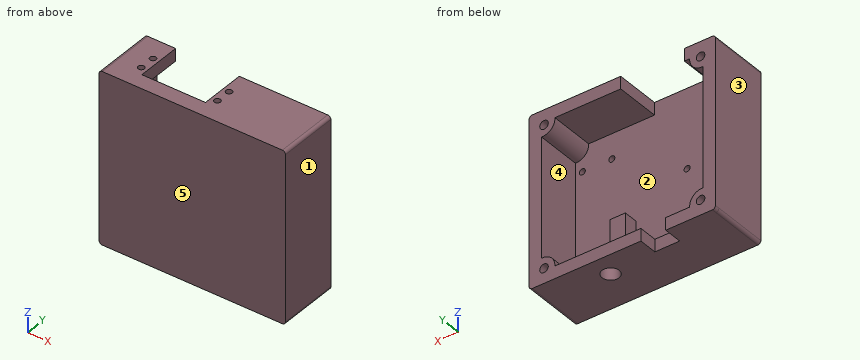
from build123d import *

# Parameters (mm, degrees)
SKETCH1_W           = 120
SKETCH1_H           = 110
BOSS_EXTRUDE1_DEPTH = 30
SKETCH2_W           = 104
SKETCH2_H           = 94
CUT_EXTRUDE1_DEPTH  = 26
FILLET1_R           = 2
CUT_EXTRUDE2_REACH  = 167.529
SKETCH3_W           = 41
SKETCH3_H           = 21
SKETCH5_R           = 2
CUT_EXTRUDE3_DEPTH  = 5
CUT_EXTRUDE4_REACH  = 167.529
SKETCH7_R           = 5.5
CUT_EXTRUDE5_REACH  = 167.529
SKETCH8_W           = 16
SKETCH8_H           = 9
SKETCH9_W           = 10
SKETCH9_H           = 32
BOSS_EXTRUDE2_DEPTH = 9
BOSS_EXTRUDE3_DEPTH = 26
BOSS_EXTRUDE4_DEPTH = 6
SKETCH11_R          = 1.95
CUT_EXTRUDE6_DEPTH  = 6
SKETCH13_R          = 2.75
CUT_EXTRUDE7_DEPTH  = 10
CUT_EXTRUDE8_REACH  = 167.529
SKETCH16_W          = 41
SKETCH16_H          = 5
BOSS_EXTRUDE5_START = 3
SKETCH21_R          = 2.75
BOSS_EXTRUDE5_DEPTH = 3


with BuildPart() as part:
    # Sketch1 → Boss-Extrude1 (new body)
    with BuildSketch(Plane(origin=(0, 0, 0), x_dir=(1, 0, 0), z_dir=(0, 1, 0))):
        with Locations((60, 55)):
            Rectangle(SKETCH1_W, SKETCH1_H)
    extrude(amount=BOSS_EXTRUDE1_DEPTH)

    # Sketch2 → Cut-Extrude1 (cut)
    with BuildSketch(Plane(origin=(0, 30, 0), x_dir=(1, 0, 0), z_dir=(0, 1, 0))):
        with Locations((60, 55)):
            Rectangle(SKETCH2_W, SKETCH2_H)
    extrude(amount=-CUT_EXTRUDE1_DEPTH, mode=Mode.SUBTRACT)

    # Fillet1
    fillet1_edges = [part.edges().sort_by_distance(p)[0] for p in [
        (112, 17, -8),
        (8, 17, -8),
        (8, 17, -102),
        (112, 17, -102),
        (0, 15, -110),
        (120, 15, -110),
        (120, 15, 0),
        (0, 15, 0),
    ]]
    fillet(fillet1_edges, radius=FILLET1_R)

    # Sketch3 → Cut-Extrude2 (cut, up to next)
    with BuildSketch(Plane.XY, mode=Mode.PRIVATE) as cut_extrude2_sk1:
        with Locations((40.5, 14.5)):
            Rectangle(SKETCH3_W, SKETCH3_H)
    cut_extrude2_tool1 = extrude(cut_extrude2_sk1.sketch, amount=-CUT_EXTRUDE2_REACH, mode=Mode.PRIVATE) & part.part
    add(cut_extrude2_tool1.solids().sort_by_distance((40.5, 14.5, 0))[0], mode=Mode.SUBTRACT)

    # Sketch5 → Cut-Extrude3 (cut)
    with BuildSketch(Plane.XY):
        with Locations((65, 8.9)):
            Circle(SKETCH5_R)
        with Locations((16, 18.9)):
            Circle(SKETCH5_R)
        with Locations((16, 8.9)):
            Circle(SKETCH5_R)
        with Locations((65, 18.9)):
            Circle(SKETCH5_R)
    extrude(amount=-CUT_EXTRUDE3_DEPTH, mode=Mode.SUBTRACT)

    # Sketch7 → Cut-Extrude4 (cut, up to next)
    with BuildSketch(Plane(origin=(0, 0, -110), x_dir=(-1, 0, 0), z_dir=(0, 0, -1)), mode=Mode.PRIVATE) as cut_extrude4_sk1:
        with Locations((-78, 19)):
            Circle(SKETCH7_R)
    cut_extrude4_tool1 = extrude(cut_extrude4_sk1.sketch, amount=-CUT_EXTRUDE4_REACH, mode=Mode.PRIVATE) & part.part
    add(cut_extrude4_tool1.solids().sort_by_distance((78, 19, -110))[0], mode=Mode.SUBTRACT)

    # Sketch8 → Cut-Extrude5 (cut, up to next)
    with BuildSketch(Plane(origin=(0, 0, -110), x_dir=(-1, 0, 0), z_dir=(0, 0, -1)), mode=Mode.PRIVATE) as cut_extrude5_sk1:
        with Locations((-40, 25.5)):
            Rectangle(SKETCH8_W, SKETCH8_H)
    cut_extrude5_tool1 = extrude(cut_extrude5_sk1.sketch, amount=-CUT_EXTRUDE5_REACH, mode=Mode.PRIVATE) & part.part
    add(cut_extrude5_tool1.solids().sort_by_distance((40, 25.5, -110))[0], mode=Mode.SUBTRACT)

    # Sketch9 → Boss-Extrude2 (add)
    with BuildSketch(Plane(origin=(0, 4, 0), x_dir=(1, 0, 0), z_dir=(0, 1, 0))):
        with Locations((78, 86)):
            Rectangle(SKETCH9_W, SKETCH9_H)
    extrude(amount=BOSS_EXTRUDE2_DEPTH)

    # Sketch10 → Boss-Extrude3 (add)
    with BuildSketch(Plane(origin=(0, 4, 0), x_dir=(1, 0, 0), z_dir=(0, 1, 0))):
        with BuildLine():
            ThreePointArc((10, 102), (8.585786438, 101.414213562), (8, 100))
            Line((8, 100), (8, 93.435688996))
            ThreePointArc((8, 93.435688996), (14.242640687, 95.757359313), (16.564311004, 102))
            Line((16.564311004, 102), (10, 102))
        make_face()
        with BuildLine():
            ThreePointArc((8, 10), (8.585786438, 8.585786438), (10, 8))
            Line((10, 8), (16.564311004, 8))
            ThreePointArc((16.564311004, 8), (14.242640687, 14.242640687), (8, 16.564311004))
            Line((8, 16.564311004), (8, 10))
        make_face()
        with BuildLine():
            ThreePointArc((110, 8), (111.414213562, 8.585786438), (112, 10))
            Line((112, 10), (112, 16.564311004))
            ThreePointArc((112, 16.564311004), (105.757359313, 14.242640687), (103.435688996, 8))
            Line((103.435688996, 8), (110, 8))
        make_face()
        with BuildLine():
            ThreePointArc((112, 100), (111.414213562, 101.414213562), (110, 102))
            Line((110, 102), (103.435688996, 102))
            ThreePointArc((103.435688996, 102), (105.757359313, 95.757359313), (112, 93.435688996))
            Line((112, 93.435688996), (112, 100))
        make_face()
    extrude(amount=BOSS_EXTRUDE3_DEPTH)

    # Sketch12 → Boss-Extrude4 (add)
    with BuildSketch(Plane.XZ):
        with BuildLine():
            Line((2, -110), (118, -110))
            ThreePointArc((118, -110), (119.414213562, -109.414213562), (120, -108))
            Line((120, -108), (120, -2))
            ThreePointArc((120, -2), (119.414213562, -0.585786438), (118, 0))
            Line((118, 0), (2, 0))
            ThreePointArc((2, 0), (0.585786438, -0.585786438), (0, -2))
            Line((0, -2), (0, -108))
            ThreePointArc((0, -108), (0.585786438, -109.414213562), (2, -110))
        make_face()
    extrude(amount=BOSS_EXTRUDE4_DEPTH)

    # Sketch11 → Cut-Extrude6 (cut)
    with BuildSketch(Plane(origin=(0, 4, 0), x_dir=(1, 0, 0), z_dir=(0, 1, 0))):
        with Locations(Location((40, 96, 0), (0, 0, 270))):
            Circle(SKETCH11_R)
        with Locations(Location((40, 51, 0), (0, 0, 270))):
            Circle(SKETCH11_R)
        with Locations(Location((88.5, 80, 0), (0, 0, 270))):
            Circle(SKETCH11_R)
        with Locations(Location((107.5, 80, 0), (0, 0, 270))):
            Circle(SKETCH11_R)
        with Locations(Location((88.5, 24, 0), (0, 0, 270))):
            Circle(SKETCH11_R)
        with Locations(Location((107.5, 24, 0), (0, 0, 270))):
            Circle(SKETCH11_R)
    extrude(amount=-CUT_EXTRUDE6_DEPTH, mode=Mode.SUBTRACT)

    # Sketch13 → Cut-Extrude7 (cut)
    with BuildSketch(Plane(origin=(0, 30, 0), x_dir=(1, 0, 0), z_dir=(0, 1, 0))):
        with Locations(Location((110.435688996, 100.435688996, 0), (0, 0, 90))):
            Circle(SKETCH13_R)
        with Locations(Location((9.564311004, 100.435688996, 0), (0, 0, 270))):
            Circle(SKETCH13_R)
        with Locations(Location((110.435688996, 9.564311004, 0), (0, 0, 270))):
            Circle(SKETCH13_R)
        with Locations(Location((9.564311004, 9.564311004, 0), (0, 0, 90))):
            Circle(SKETCH13_R)
    extrude(amount=-CUT_EXTRUDE7_DEPTH, mode=Mode.SUBTRACT)

    # Sketch16 → Cut-Extrude8 (cut, up to next)
    with BuildSketch(Plane.XY, mode=Mode.PRIVATE) as cut_extrude8_sk1:
        with Locations((40.5, 27.5)):
            Rectangle(SKETCH16_W, SKETCH16_H)
    cut_extrude8_tool1 = extrude(cut_extrude8_sk1.sketch, amount=-CUT_EXTRUDE8_REACH, mode=Mode.PRIVATE) & part.part
    add(cut_extrude8_tool1.solids().sort_by_distance((40.5, 27.5, 0))[0], mode=Mode.SUBTRACT)

    # Sketch21 → Boss-Extrude5 (add)
    # profile 1 of 2: a face of its own
    with BuildSketch(Plane(origin=(0, 30, 0), x_dir=(1, 0, 0), z_dir=(0, 1, 0)).offset(BOSS_EXTRUDE5_START)):
        with BuildLine():
            ThreePointArc((112, 16.564311004), (105.757359313, 14.242640687), (103.435688996, 8))
            Line((103.435688996, 8), (61, 8))
            Line((61, 8), (61, 0))
            Line((61, 0), (118, 0))
            ThreePointArc((118, 0), (119.414213562, 0.585786438), (120, 2))
            Line((120, 2), (120, 108))
            ThreePointArc((120, 108), (119.414213562, 109.414213562), (118, 110))
            Line((118, 110), (48, 110))
            Line((48, 110), (48, 102))
            Line((48, 102), (103.435688996, 102))
            ThreePointArc((103.435688996, 102), (105.757359313, 95.757359313), (112, 93.435688996))
            Line((112, 93.435688996), (112, 16.564311004))
        make_face()
        with Locations((110.435688996, 9.564311004)):
            Circle(SKETCH21_R, mode=Mode.SUBTRACT)
        with Locations((110.435688996, 100.435688996)):
            Circle(SKETCH21_R, mode=Mode.SUBTRACT)
    # profile 2 of 2: a face of its own
    with BuildSketch(Plane(origin=(0, 30, 0), x_dir=(1, 0, 0), z_dir=(0, 1, 0)).offset(BOSS_EXTRUDE5_START)):
        with BuildLine():
            Line((8, 16.564311004), (8, 93.435688996))
            ThreePointArc((8, 93.435688996), (14.242640687, 95.757359313), (16.564311004, 102))
            Line((16.564311004, 102), (32, 102))
            Line((32, 102), (32, 110))
            Line((32, 110), (2, 110))
            ThreePointArc((2, 110), (0.585786438, 109.414213562), (0, 108))
            Line((0, 108), (0, 2))
            ThreePointArc((0, 2), (0.585786438, 0.585786438), (2, 0))
            Line((2, 0), (20, 0))
            Line((20, 0), (20, 8))
            Line((20, 8), (16.564311004, 8))
            ThreePointArc((16.564311004, 8), (14.242640687, 14.242640687), (8, 16.564311004))
        make_face()
        with Locations((9.564311004, 9.564311004)):
            Circle(SKETCH21_R, mode=Mode.SUBTRACT)
        with Locations((9.564311004, 100.435688996)):
            Circle(SKETCH21_R, mode=Mode.SUBTRACT)
    extrude(amount=-BOSS_EXTRUDE5_DEPTH)


solid = part.part
The listing builds one solid part. Answer for the finished solid, in the listing's coordinates (mm). Face numbers are marked on the shaded views. A direction names the side the tool comes from. Give positions to 0.01 mm unless a question says otherwise; leave off trailing zeros. Write each loop counter-clockwise with the first axis right and the second up, starting at its lowest first coordinate (ties: lowest second). Pieces come first, ordered by that corner, then holes.
1) Section D-D (z = -91.5) is taken. Write down the section's boundary in (x, y).
2) Given P1, Ø6, axis at x = 40, z = -96, coming from the +Y side; P2, Ø1.5, axis at x = 25, y = 12.5, coming from the +Z side; P3, Ø2, axis at x = 65, y = 8, coming from the +Z side, each flat-ended and moving along its own axis, determine where each tip first touches the part or whether it passes through.
3) For a pull along X with two mould halves and no side action, classify the marked faces 1, 2 and 3 as pulls with the +X half, pulls with the -X half, needs draft (parallel to the pull), parting line crosses it, or undercut.
4) Section A-A (z = -24) is taken. Write down the section's boundary in (x, y).
5) Section C-C (y = 28.5) is taken. Write down the section's boundary in (x, z), and give its area (3 significant figures).
6) A tool of negligible diameter and unlimited length cuts with its end or side. For the marked faces 4 and 5, from which of +Z, -Z, +X, -X, +Y, -Y can it reach the whole face along a straight path? Write none if from no direction.
7) Find the intervals of material crossed by L1, parallel to X at y = -0.7, z = -80; L2, parallel to X at y = 0.65, z = -96; L3, parallel to Z at x = 99.5, y = 9.5, in increasing order.
8) Section B-B (x = 88.5) is taken. Write down the section's boundary in (y, z), and give its area (3 significant figures).
Response:
1. outline: (0, -6) - (120, -6) - (120, 33) - (112, 33) - (112, 4) - (83, 4) - (83, 13) - (73, 13) - (73, 4) - (8, 4) - (8, 33) - (0, 33) - close
2. P1: stops at y = 4
2. P2: stops at z = -102
2. P3: stops at z = -5
3. face 1: pulls with the +X half
3. face 2: undercut
3. face 3: pulls with the -X half
4. outline: (0, -6) - (120, -6) - (120, 33) - (112, 33) - (112, 4) - (109.45, 4) - (109.45, -2) - (105.55, -2) - (105.55, 4) - (90.45, 4) - (90.45, -2) - (86.55, -2) - (86.55, 4) - (8, 4) - (8, 33) - (0, 33) - close
5. outline: (0, -108) arc R2 ccw to (2, -110) - (32, -110) - (32, -102) - (16.56, -102) arc R8 ccw to (8, -93.44) - (8, -16.56) arc R8 ccw to (16.56, -8) - (20, -8) - (20, 0) - (2, 0) arc R2 ccw to (0, -2) - close; (48, -110) - (118, -110) arc R2 ccw to (120, -108) - (120, -2) arc R2 ccw to (118, 0) - (61, 0) - (61, -8) - (103.44, -8) arc R8 ccw to (112, -16.56) - (112, -93.44) arc R8 ccw to (103.44, -102) - (48, -102) - close; hole circle Ø5.5 at (9.56, -100.44); hole circle Ø5.5 at (9.56, -9.56); hole circle Ø5.5 at (110.44, -100.44); hole circle Ø5.5 at (110.44, -9.56)
5. area: 3,110 mm2
6. face 4: +Y
6. face 5: +Z, -Z, +X, -X, -Y
7. L1: x = 0 to 86.55, 90.45 to 105.55, 109.45 to 120
7. L2: x = 0 to 38.05, 41.95 to 120
7. L3: z = -110 to -102, -8 to 0
8. outline: (-6, -110) - (33, -110) - (33, -102) - (4, -102) - (4, -81.95) - (-2, -81.95) - (-2, -78.05) - (4, -78.05) - (4, -25.95) - (-2, -25.95) - (-2, -22.05) - (4, -22.05) - (4, -8) - (33, -8) - (33, 0) - (-6, 0) - close
8. area: 1,520 mm2
